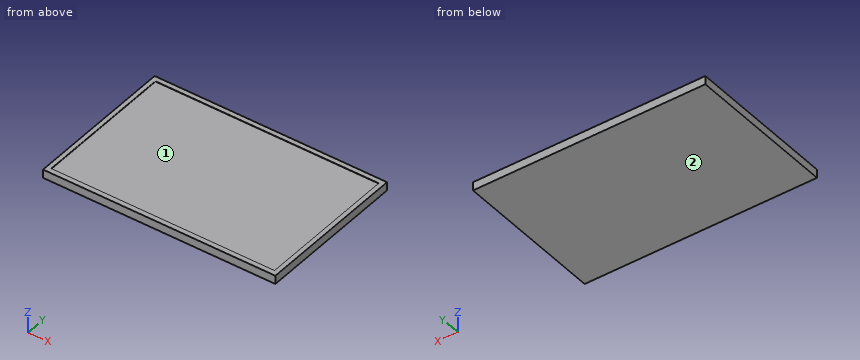
from build123d import *

# Parameters (mm, degrees)
F0_W          = 220
F0_H          = 139
F1_DEPTH      = 8
F0_W_2        = 229
F0_H_2        = 149
F2_DEPTH      = 0.3
F2_DEPTH_BACK = 8


with BuildPart() as f1:
    # F0 (on Top) → F1 (new body)
    with BuildSketch(Plane.XY):
        Rectangle(F0_W, F0_H)
    extrude(amount=-F1_DEPTH)

    # F0 (on Top) → F2 (join, two sides)
    with BuildSketch(Plane.XY) as f2_sk:
        Rectangle(F0_W_2, F0_H_2)
        Rectangle(F0_W, F0_H, mode=Mode.SUBTRACT)
    extrude(amount=F2_DEPTH)
    extrude(f2_sk.sketch, amount=-F2_DEPTH_BACK)


solid = f1.part
Input: part model. Units: mm. Frame: model coordinates. Face numbers are marked on the shaded views. Coordinates: 2 decimals unless noted, no trailing zeros. Loops run counter-clockwise (first coordinate to the right, second up) from the corner with the lowest first, then second, coordinate; pieces in that order, holes last. Notation, with made-up numbers: (-30.5, 36) -> (13.5, 36) arc R23 ccw to (13.5, 56) -> close; hole circle Ø9 at (30, 19). An arc over 180 degrees is marked (long way). Write item = value, one per line. Start each with the question number.
Item 1: Mould query, pull axis X, two halves, no side actions, for the marked faces 1 and 2. Classes: pulls with the +X half, pulls with the -X half, needs draft (parallel to the pull), parting line crosses it, or undercut.
Item 2: Cut plane B-B, the plane y = 25. Return loops of the section in (x, z).
Item 3: Cut plane A-A, the plane x = 26. Return loops of the section in (y, z), plus the area to 4 significant figures.
Item 4: Material intervals for line 1 (Z direction, x = 78, y = -62), sorted ascending.
Item 5: First-contact query: P1, Ø1.5, axis at x = 20, y = 2.5, coming from the +Z side. Flat tip, straight axial feed; report the tip coordinate or a pass-through.
Ans:
q1.face_1 = undercut
q1.face_2 = needs draft
q2.outline = (-114.5, -8) -> (114.5, -8) -> (114.5, 0.3) -> (110, 0.3) -> (110, 0) -> (-110, 0) -> (-110, 0.3) -> (-114.5, 0.3) -> close
q3.outline = (-74.5, -8) -> (74.5, -8) -> (74.5, 0.3) -> (69.5, 0.3) -> (69.5, 0) -> (-69.5, 0) -> (-69.5, 0.3) -> (-74.5, 0.3) -> close
q3.area = 1,195 mm²
q4.line_1 = -8 to 0
q5.P1 = 0
